```python
from build123d import *

# Parameters (mm, degrees)
F1_DEPTH = 3.9878


with BuildPart() as f1:
    # F0 (on Top) → F1 (new body)
    with BuildSketch(Plane.XY):
        with BuildLine():
            Line((-38.1, 0), (0, 0))
            Line((0, 0), (0, -56.261))
            ThreePointArc((0, -56.261), (44.596761, -35.22038), (71.12, 6.35))
            ThreePointArc((71.12, 6.35), (67.181938, 39.92176), (38.1, 57.15))
            ThreePointArc((38.1, 57.15), (14.508681, 50.302599), (0, 30.48))
            Line((0, 30.48), (0, 6.35))
            Line((0, 6.35), (-38.1, 6.35))
            Line((-38.1, 6.35), (-38.1, 0))
        make_face()
    extrude(amount=F1_DEPTH)


solid = f1.part
```
Build history of the part. All positions in model axes, mm. A direction names the side the tool comes from. Round coordinates to 2 decimals unless told otherwise and drop trailing zeros. Write each loop counter-clockwise with the first axis right and the second up, starting at its lowest first coordinate (ties: lowest second). Pieces come first, ordered by that corner, then holes. Notation, with made-up numbers: (10, 61) - (33, 61) arc R34 ccw to (33, 92) - close; hole circle Ø10 at (42, 55). An arc over 180 degrees is marked (long way). Write each question's results on one line, items separated by ' | '. Start each with the question number.
Item 1: Which spindle directions (+Z, -Z, +X, -X, +Y, -Y) get a long thin tool onto all of the face, cutting with end or side? Do faces 1 (the face through (0, -28, 2)), 2 (the face through (-19, 6.35, 2)), 3 (the face through (29, 1, 3.988)). Say none if no direction does.
Item 2: Saw through at C-C (y = -10.5). Write the cut outline in (x, z), and give its area (3 significant figures).
Item 3: Saw through at A-A (z = 2.8). Write the cut outline in (x, y).
Item 4: Wall check: L1, parallel to Y at x = -14, z = 1.45; L2, parallel to Y at x = 35, z = 3.3; L3, parallel to X at y = -22.5, z = 3.4. Give the ranges that are in metal, low to high. Write a range as [from, to].
Item 5: Saw through at B-B (x = -25.5). Write the cut outline in (y, z).
Item 6: Drop flat-ended pins along their axis: P1, Ø1, axis at x = 53.5, z = 2.5, coming from the +Y side; P2, Ø1, axis at y = -31, z = 2, coming from the +X side. Give the stop position or say it passes through.
Results are:
1) face 1: +Z, -Z, -X, -Y | face 2: +Z, -Z, -X, +Y | face 3: +Z, +X, -X, +Y, -Y
2) outline: (0, 0) - (64.2, 0) - (64.2, 3.99) - (0, 3.99) - close | area: 256 mm²
3) outline: (-38.1, 0) - (0, 0) - (0, -56.26) arc R88.9 ccw to (71.12, 6.35) arc R38.1 ccw to (38.1, 57.15) arc R38.1 ccw to (0, 30.48) - (0, 6.35) - (-38.1, 6.35) - close
4) L1: y = [0, 6.35] | L2: y = [-42.57, 57.17] | L3: x = [0, 56.47]
5) outline: (0, 0) - (6.35, 0) - (6.35, 3.99) - (0, 3.99) - close
6) P1: stops at y = 52.86 | P2: stops at x = 49.56
